The model under review builds one solid part; all positions refer to its coordinate system, in mm. Round coordinates to 2 decimals unless told otherwise and drop trailing zeros. Loops run counter-clockwise (first coordinate to the right, second up) from the corner with the lowest first, then second, coordinate; pieces in that order, holes last. Notation, with made-up numbers: (53, -33) -> (86, -33) arc R25 ccw to (86, -1) -> close; hole circle Ø1 at (57, -33). An arc over 180 degrees is marked (long way). Use a Markdown table: item, result. Add a question column.
1) Consider section C-C on x = 311. Give the boundary of the cut face in (y, z), plus the area to 3 significant figures.
2) Consider section A-A on x = 76.2. Give the boundary of the cut face in (y, z), plus the area to 3 significant figures.
3) Consider section B-B on y = -44.25. State how many separate pieces and enclosed holes the cut face has, plus the area to 3 significant figures.
4) Wall thickness on probe 1 along Z at (x, y) = (203.2, -47); probe 2 along Z at (x, y) = (432, -41); probe 3 along Z at (x, y) = (123.5, -38.25): over which ranges is each line inside the solid? List them lowest first.
5) Insertion check: pin 1 (7.5 mm diameter, centred on x = 482.6, z = 122.48, fed in from -Y); pin 2 (8 mm diameter, centred on x = 330.5, z = 69.5, fed in from +Y); pin 3 (5 mm diameter, centred on x = 384, z = 125.5, fed in from +Y). Each pin has a flat end and moves straight along its axis. Give the tip position at first contact, or say it passes through.
from build123d import *

# Parameters (mm, degrees)
F1_DEPTH       = 609.6
F3_D           = 10.71626
F6_D           = 12.7254
F6_CBORE_D     = 15.875
F6_CBORE_DEPTH = 2.54


with BuildPart() as f1:
    # F0 (on Right) → F1 (new body)
    with BuildSketch(Plane.YZ):
        Polygon((-32.1863732547, 224.0715666294), (-51.2363732547, 224.0715666294), (-51.2363732547, 20.8715666294), (-32.1863732547, 20.8715666294), (-32.1863732547, 60.9400666294), (-38.9173732547, 54.2090666294), (-38.9173732547, 62.1465666294), (-39.1713732547, 62.1465666294), (-39.1713732547, 81.1965666294), (-38.9173732547, 81.1965666294), (-38.9173732547, 89.1467666294), (-32.1863732547, 82.4157666294), (-32.1863732547, 162.5400666294), (-38.9173732547, 155.8090666294), (-38.9173732547, 163.7465666294), (-39.1713732547, 163.7465666294), (-39.1713732547, 182.7965666294), (-38.9173732547, 182.7965666294), (-38.9173732547, 190.7467666294), (-32.1863732547, 184.0157666294), align=None)
    extrude(amount=F1_DEPTH)

    # F3 (through all)
    with Locations(Plane.XZ.offset(51.2363732547)):
        with Locations((50.8, 200.2717666294), (203.2, 200.2717666294), (406.4, 200.2717666294), (558.8, 200.2717666294), (558.8, 44.6713666294), (406.4, 44.6713666294), (203.2, 44.6713666294), (50.8, 44.6713666294)):
            Hole(F3_D / 2)

    # F6 (through all)
    with Locations(Plane(origin=(0, -32.1863732547, 0), x_dir=(-1, 0, 0), z_dir=(0, 1, 0))):
        with Locations((-584.2, 122.4779166294), (-533.4, 122.4779166294), (-482.6, 122.4779166294), (-381, 122.4779166294), (-330.2, 122.4779166294), (-279.4, 122.4779166294), (-228.6, 122.4779166294), (-177.8, 122.4779166294), (-127, 122.4779166294), (-76.2, 122.4779166294), (-431.8, 122.4779166294), (-25.4, 122.4779166294)):
            CounterBoreHole(F6_D / 2, F6_CBORE_D / 2, F6_CBORE_DEPTH)


solid = f1.part
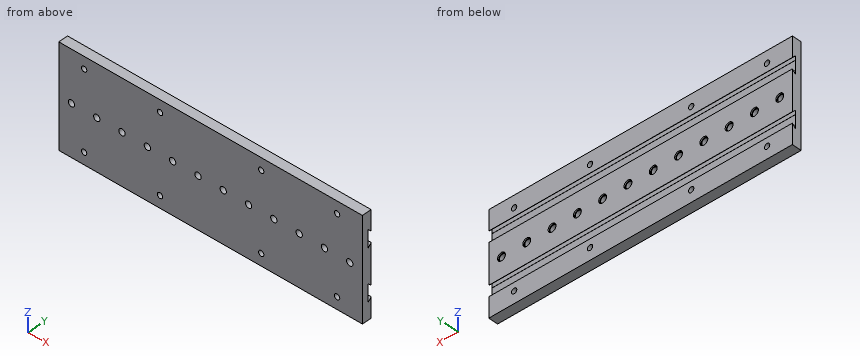
Result set:
| question | item | result |
|---|---|---|
| 1 | outline | (-51.24, 20.87) -> (-32.19, 20.87) -> (-32.19, 60.94) -> (-38.92, 54.21) -> (-38.92, 62.15) -> (-39.17, 62.15) -> (-39.17, 81.2) -> (-38.92, 81.2) -> (-38.92, 89.15) -> (-32.19, 82.42) -> (-32.19, 162.54) -> (-38.92, 155.81) -> (-38.92, 163.75) -> (-39.17, 163.75) -> (-39.17, 182.8) -> (-38.92, 182.8) -> (-38.92, 190.75) -> (-32.19, 184.02) -> (-32.19, 224.07) -> (-51.24, 224.07) -> close |
| 1 | area | 3,480 mm2 |
| 2 | outline | (-51.24, 20.87) -> (-32.19, 20.87) -> (-32.19, 60.94) -> (-38.92, 54.21) -> (-38.92, 62.15) -> (-39.17, 62.15) -> (-39.17, 81.2) -> (-38.92, 81.2) -> (-38.92, 89.15) -> (-32.19, 82.42) -> (-32.19, 114.54) -> (-34.73, 114.54) -> (-34.73, 116.12) -> (-51.24, 116.12) -> close; (-51.24, 128.84) -> (-34.73, 128.84) -> (-34.73, 130.42) -> (-32.19, 130.42) -> (-32.19, 162.54) -> (-38.92, 155.81) -> (-38.92, 163.75) -> (-39.17, 163.75) -> (-39.17, 182.8) -> (-38.92, 182.8) -> (-38.92, 190.75) -> (-32.19, 184.02) -> (-32.19, 224.07) -> (-51.24, 224.07) -> close |
| 2 | area | 3,230 mm2 |
| 3 | separate pieces | 1 |
| 3 | enclosed holes | 20 |
| 3 | area | 122,000 mm2 |
| 4 | probe 1 | 20.87 to 39.31, 50.03 to 194.91, 205.63 to 224.07 |
| 4 | probe 2 | 20.87 to 116.12, 128.84 to 224.07 |
| 4 | probe 3 | 20.87 to 54.88, 88.48 to 117.16, 127.79 to 156.48, 190.08 to 224.07 |
| 5 | pin 1 | through |
| 5 | pin 2 | y = -39.17 |
| 5 | pin 3 | y = -34.73 |
